Here's the drawing with two shaded views (mm, measured from the low corner). I have some questions. A direction names the side the tool comes from. Coordinates: 2 decimals unless noted, no trailing zeros. Write each loop counter-clockwise with the first axis right and the second up, starting at its lowest first coordinate (ties: lowest second). Pieces come first, ordered by that corner, then holes.
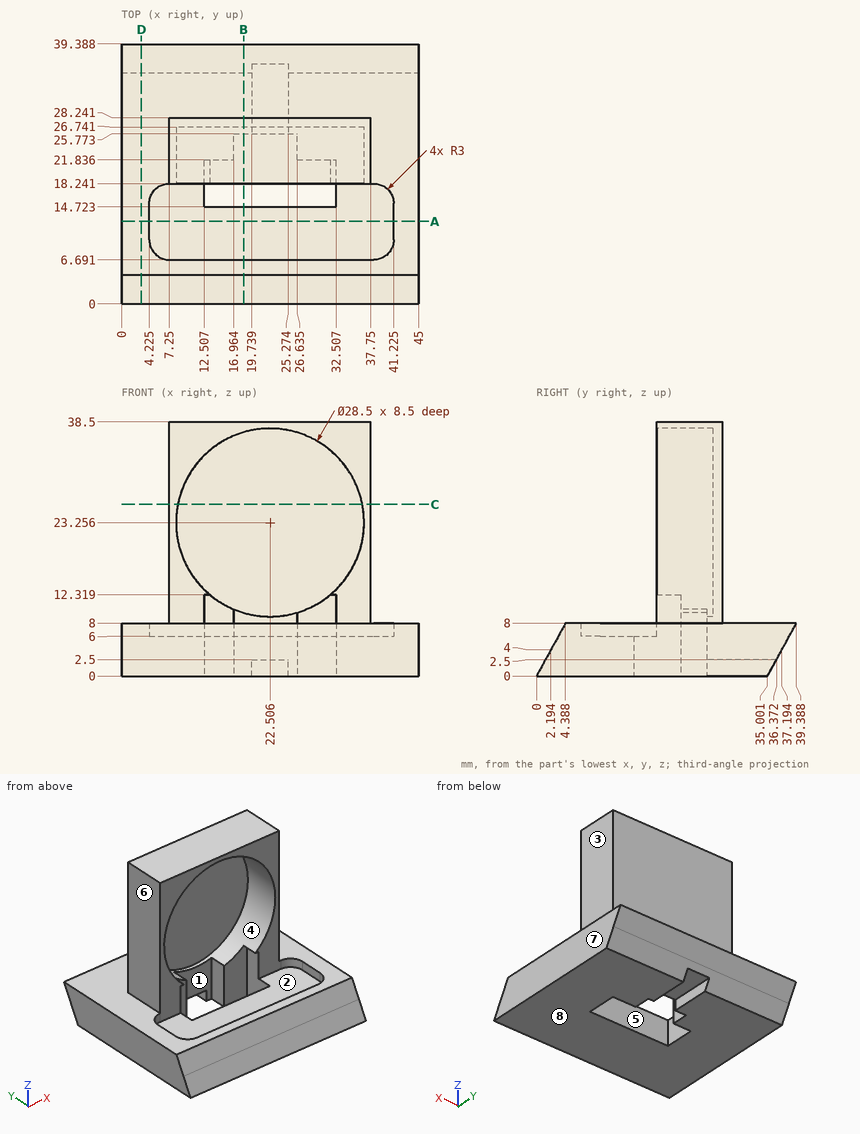
1. If we section it at C-C, the plane z = 26: List the corners of the cut face in (x, y) for me.
2. We'd pull the mould along X, two halves only. Please class the marked faces 5, 6, 7 and 8: released by +X, released by -X, zero draft, split by the parting line, or undercut.
3. If I drill on L1, parallel to X at y = 25, z = 7 (1 decimal); L2, parallel to X at y = 20, z = 10.5; L3, parallel to Y at x = 14, z = 27, over which ranges is the centre line in solid material (lowest first)?
4. If we section it at B-B, the plane x = 18.5: List the corners of the cut face in (y, z) for me (1 decimal).
5. If we section it at A-A, the plane y = 12.5: List the corners of the cut face in (x, z) for me (1 decimal), plus the area to 3 significant figures.
6. I'm going to push flat-ended pins straight in: P1, Ø2, axis at x = 14.5, z = 6.5, coming from the -Y side; P2, Ø0.7, axis at x = 13, y = 20.5, coming from the -Z side; P3, Ø3, axis at y = 23, z = 16, coming from the +X side. Where does each tip first touch, or does it pass through?
7. If we section it at D-D, the plane x = 3: List the corners of the cut face in (y, z) for me (1 decimal).
8. Which directions (+Z, -Z, +X, -X, +Y, -Y) give clear straight access to the entire face, cutting with the end or side of a thin tool? Please do the marked faces 1, 2, 3 and 4.
Answers:
1. outline: (7.25, 18.24) - (8.52, 18.24) - (8.52, 26.74) - (36.49, 26.74) - (36.49, 18.24) - (37.75, 18.24) - (37.75, 28.24) - (7.25, 28.24) - close
2. face 5: undercut
2. face 6: released by -X
2. face 7: released by +X
2. face 8: zero draft
3. L1: x = 0 to 17, 26.6 to 45
3. L2: x = 7.25 to 12.51, 32.51 to 37.75
3. L3: y = 26.74 to 28.24
4. outline: (0, 0) - (14.7, 0) - (14.7, 6) - (6.7, 6) - (6.7, 8) - (4.4, 8) - (2.2, 4) - close; (18.2, 36.9) - (26.7, 36.9) - (26.7, 9.6) - (25.8, 9.6) - (25.8, 0) - (35, 0) - (37.2, 4) - (39.4, 8) - (28.2, 8) - (28.2, 38.5) - (18.2, 38.5) - close
5. outline: (0, 0) - (45, 0) - (45, 8) - (41.2, 8) - (41.2, 6) - (4.2, 6) - (4.2, 8) - (0, 8) - close
5. area: 286 mm2
6. P1: stops at y = 3.02
6. P2: stops at z = 12.32
6. P3: stops at x = 37.75
7. outline: (0, 0) - (35, 0) - (37.2, 4) - (39.4, 8) - (4.4, 8) - (2.2, 4) - close
8. face 1: -Z
8. face 2: +Z
8. face 3: +Z, +X, +Y, -Y
8. face 4: -Y
